Can you work these out from the model? Positions are in its coordinate system, mm. A direction names the side the tool comes from. Coordinates: 2 decimals unless noted, no trailing zeros. Order: outer loops, then holes, each group sorted by start corner. A loop starts at its lowest first (then second) coordinate and runs counter-clockwise, first axis right, second up. Notation, with made-up numbers: (34.5, -6.5) -> (53.5, -6.5) arc R21 cw to (53.5, 25.5) -> close; hole circle Ø11 at (-10, 57.5). An arc over 180 degrees is marked (long way). Answer in a Markdown table with one row per item.
```python
from build123d import *

# Parameters (mm, degrees)
SKETCH1_R           = 3
BOSS_EXTRUDE1_DEPTH = 5


with BuildPart() as part:
    # Sketch1 → Boss-Extrude1 (new body)
    with BuildSketch(Plane.XY):
        with BuildLine():
            ThreePointArc((195, -42), (203.5, -33.5), (195, -25))
            Line((195, -25), (188.821366739, -25))
            Line((188.821366739, -25), (127.15841734, 4.510125784))
            ThreePointArc((127.15841734, 4.510125784), (122.334675132, 4.230371538), (120, 0))
            Line((120, 0), (120, -13))
            ThreePointArc((120, -13), (115.606601718, -23.606601718), (105, -28))
            Line((105, -28), (20, -28))
            ThreePointArc((20, -28), (9.393398282, -23.606601718), (5, -13))
            Line((5, -13), (5, 0))
            ThreePointArc((5, 0), (0, 5), (-5, 0))
            Line((-5, 0), (-5, -27))
            ThreePointArc((-5, -27), (-0.606601734, -37.606601701), (9.999999954, -42))
            Line((9.999999954, -42), (195, -42))
        make_face()
        with BuildLine():
            Line((196.651752124, -28.780708218), (196.661737841, -28.752177599))
            Line((196.661737841, -28.752177599), (197.15841734, -28.989874216))
            ThreePointArc((197.15841734, -28.989874216), (193.092046793, -38.121657123), (196.651752124, -28.780708218))
        make_face(mode=Mode.SUBTRACT)
        with BuildLine():
            Line((130, -7.902630298), (165.725847138, -25))
            Line((165.725847138, -25), (145, -25))
            ThreePointArc((145, -25), (134.393398282, -20.606601718), (130, -10))
            Line((130, -10), (130, -7.902630298))
        make_face(mode=Mode.SUBTRACT)
        with Locations((125, 0)):
            Circle(SKETCH1_R, mode=Mode.SUBTRACT)
        Circle(SKETCH1_R, mode=Mode.SUBTRACT)
    extrude(amount=BOSS_EXTRUDE1_DEPTH)


solid = part.part
```
(1) Suppose I cut it at A-A (x = 125). Please give me the cut outline in (y, z), and give its area (3 significant figures).
Response values:
| item | result |
|---|---|
| outline | (-42, 0) -> (-3, 0) -> (-3, 5) -> (-42, 5) -> close; (3, 0) -> (5, 0) -> (5, 5) -> (3, 5) -> close |
| area | 205 mm2 |
(2) I need wall thicknesses on line 1 (Y direction, x = 125, z = 1.9); line 2 (X direction, y = -10.5, z = 2.3); line 3 (X direction, y = -12, z = 1). Which ranges of each line are inside material? Lowest first, please. Write a range as [from, to].
Response values:
| item | result |
|---|---|
| line 1 | [-42, -3], [3, 5] |
| line 2 | [-5, 5], [120, 130.01], [135.43, 158.52] |
| line 3 | [-5, 5], [120, 130.13], [138.56, 161.66] |
(3) On a 3-axis mill with a long thin cutter (end or side, diameter ignored), from which of +Z, -Z, +X, -X, +Y, -Y can I reach the whole of each face in a straight line? I mean faces 1 (the flat face through (63, -28, 2)), 2 (the flat face through (98, -29, 5)), 3 (the flat face through (147.61, -16.33, 2.46)). Say none if no direction works.
Response values:
| item | result |
|---|---|
| face 1 | +Z, -Z, +Y |
| face 2 | +Z, +X, -X, +Y, -Y |
| face 3 | +Z, -Z |
(4) We'd pull the mould along X, two halves only. Please class faces 4 (the cylindrical face through (9.51, -23.72, 2.46)), 5 (the flat face through (158.42, -10.45, 2.46)), 6 (the flat face through (98, -29, 0)): +X half, -X half, draft (parallel to the pull), parting line (faces both ways), or undercut.
Response values:
| item | result |
|---|---|
| face 4 | undercut |
| face 5 | +X half |
| face 6 | draft |
(5) Suppose I cut it at C-C (z = 0.95). Count the separate pieces of the cut face and the enclosed holes in it, and give its area (3 significant figures).
Response values:
| item | result |
|---|---|
| separate pieces | 1 |
| enclosed holes | 4 |
| area | 4,230 mm2 |
(6) Will these pins go through, and if not, where does the flat tip stop? pin 1 Ø1.5 at (x, z) = (158, 1.5) entering from +Y; pin 2 Ø16 at (x, y) = (195, -33.5) entering from -Z; pin 3 Ø1.5 at (x, z) = (58, 3) entering from +Y; pin 4 Ø2.5 at (x, z) = (193, 3) entering from +Y.
Response values:
| item | result |
|---|---|
| pin 1 | y = -9.89 |
| pin 2 | z = 0 |
| pin 3 | y = -28 |
| pin 4 | y = -25 |
(7) Suppose I cut it at B-B (y = -33.5). Please give me the cut outline in (x, z).
Response values:
| item | result |
|---|---|
| outline | (-3.52, 0) -> (190, 0) -> (190, 5) -> (-3.52, 5) -> close; (200, 0) -> (203.5, 0) -> (203.5, 5) -> (200, 5) -> close |
(8) Suppose I cut it at D-D (y = -21.5). Please give me the cut outline in (x, z).
Response values:
| item | result |
|---|---|
| outline | (-5, 0) -> (7.64, 0) -> (7.64, 5) -> (-5, 5) -> close; (117.36, 0) -> (135.37, 0) -> (135.37, 5) -> (117.36, 5) -> close; (158.41, 0) -> (181.51, 0) -> (181.51, 5) -> (158.41, 5) -> close |
